Check sheet for the modelled part. Datum: model origin and axes. Units: mm. Coordinates: 2 decimals unless noted, no trailing zeros. Loops run counter-clockwise (first coordinate to the right, second up) from the corner with the lowest first, then second, coordinate; pieces in that order, holes last.
```python
from build123d import *

# Parameters (mm, degrees)
SKETCH_1_W             = 200
SKETCH_1_H             = 65
SKETCH_1_R             = 2.1
SKETCH_1_W_2           = 80
SKETCH_1_H_2           = 50
EXTRUDE_1_DEPTH        = 3
SKETCH_2_R             = 1.6
CUT_EXTRUDE_1454_DEPTH = 130.673628776
SKETCH_3_R             = 1.6
CUT_EXTRUDE_2001_DEPTH = 130.673628776
FILLET_1_R             = 10


with BuildPart() as part:
    # 草图1 → 凸台-拉伸1 (new body)
    # profile 1 of 2: a face of its own
    with BuildSketch(Plane(origin=(0, 0, 0), x_dir=(1, 0, 0), z_dir=(0, 1, 0))):
        Rectangle(SKETCH_1_W, SKETCH_1_H)
        with Locations(Location((85, -12.5, 0), (0, 0, 270))):
            Circle(SKETCH_1_R, mode=Mode.SUBTRACT)
        with Locations(Location((-85, -12.5, 0), (0, 0, 270))):
            Circle(SKETCH_1_R, mode=Mode.SUBTRACT)
        with Locations(Location((-85, 22.5, 0), (0, 0, 270))):
            Circle(SKETCH_1_R, mode=Mode.SUBTRACT)
        with Locations(Location((85, 22.5, 0), (0, 0, 270))):
            Circle(SKETCH_1_R, mode=Mode.SUBTRACT)
    # profile 2 of 2: a face of its own
    with BuildSketch(Plane(origin=(0, 0, 0), x_dir=(1, 0, 0), z_dir=(0, 1, 0))):
        with Locations((0, -57.5)):
            Rectangle(SKETCH_1_W_2, SKETCH_1_H_2)
    extrude(amount=EXTRUDE_1_DEPTH)

    # 草图2 → Cut-Extrude 1454 (cut, through all)
    with BuildSketch(Plane(origin=(0, 3, 0), x_dir=(1, 0, 0), z_dir=(0, 1, 0))):
        with Locations(Location((-60, 17.5, 0), (0, 0, 270))):
            Circle(SKETCH_2_R)
        with Locations(Location((-60, -17.5, 0), (0, 0, 270))):
            Circle(SKETCH_2_R)
        with Locations(Location((60, -17.5, 0), (0, 0, 270))):
            Circle(SKETCH_2_R)
        with Locations(Location((60, 17.5, 0), (0, 0, 270))):
            Circle(SKETCH_2_R)
    extrude(amount=-CUT_EXTRUDE_1454_DEPTH, mode=Mode.SUBTRACT)

    # 草图3 → Cut-Extrude 2001 (cut, through all)
    with BuildSketch(Plane(origin=(0, 3, 0), x_dir=(1, 0, 0), z_dir=(0, 1, 0))):
        with Locations(Location((-22.773937698, -58.5, 0), (0, 0, 270))):
            Circle(SKETCH_3_R)
        with Locations(Location((24.226062302, -58.5, 0), (0, 0, 90))):
            Circle(SKETCH_3_R)
        with Locations(Location((24.226062302, -76.5, 0), (0, 0, 270))):
            Circle(SKETCH_3_R)
        with Locations(Location((-22.773937698, -76.5, 0), (0, 0, 90))):
            Circle(SKETCH_3_R)
        with Locations(Location((-6.273937698, -59.5, 0), (0, 0, 270))):
            Circle(SKETCH_3_R)
        with Locations(Location((7.726062302, -59.5, 0), (0, 0, 90))):
            Circle(SKETCH_3_R)
        with Locations(Location((7.726062302, -75.5, 0), (0, 0, 270))):
            Circle(SKETCH_3_R)
        with Locations(Location((-6.273937698, -75.5, 0), (0, 0, 90))):
            Circle(SKETCH_3_R)
    extrude(amount=-CUT_EXTRUDE_2001_DEPTH, mode=Mode.SUBTRACT)

    # 圆角1
    fillet_1_edges = [part.edges().sort_by_distance(p)[0] for p in [
        (40, 1.5, 32.5),
        (-40, 1.5, 32.5),
    ]]
    fillet(fillet_1_edges, radius=FILLET_1_R)


solid = part.part
```
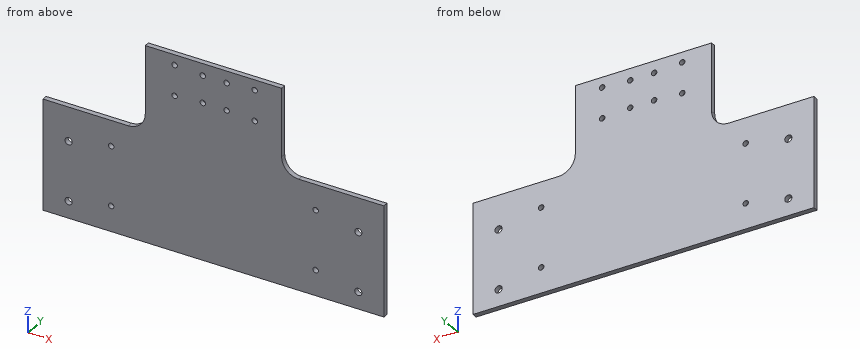
1) Section check C-C on y = 1.75. Give the number of separate pieces and of enclosed holes in the cut face, plus the area to 3 significant figures.
Answer sheet:
separate pieces: 1
enclosed holes: 16
area: 16,900 mm2
2) Section check D-D on x = 81. Enter the section's corners in (y, z).
Answer sheet:
outline: (0, -32.5) - (3, -32.5) - (3, 32.5) - (0, 32.5) - close
3) Section check B-B on z = 12.5. Enter the section's corners in (x, y).
Answer sheet:
outline: (-100, 0) - (-87.1, 0) - (-87.1, 3) - (-100, 3) - close; (-82.9, 0) - (82.9, 0) - (82.9, 3) - (-82.9, 3) - close; (87.1, 0) - (100, 0) - (100, 3) - (87.1, 3) - close
4) Scan lines: line 1 (X direction, y = 1.15, z = 12.5); line 2 (X direction, y = 1.85, z = 58.5); line 3 (X direction, y = 1.45, z = 75.5). Record each from-to range of solid material in increasing order.
Answer sheet:
line 1: x = -100 to -87.1, -82.9 to 82.9, 87.1 to 100
line 2: x = -40 to -24.37, -21.17 to -7.52, -5.02 to 6.48, 8.98 to 22.63, 25.83 to 40
line 3: x = -40 to -24.02, -21.52 to -7.87, -4.67 to 6.13, 9.33 to 22.98, 25.48 to 40
5) Section check A-A on x = -85. Enter the section's corners in (y, z).
Answer sheet:
outline: (0, -32.5) - (3, -32.5) - (3, -24.6) - (0, -24.6) - close; (0, -20.4) - (3, -20.4) - (3, 10.4) - (0, 10.4) - close; (0, 14.6) - (3, 14.6) - (3, 32.5) - (0, 32.5) - close
6) Depth check by flat-ended pin: pin 1 (1.5 mm diameter, centred on x = -76, y = 1.5, fed in from +Z). Enter the tip coordinate at first touch or a pass-through.
Answer sheet:
pin 1: stops at z = 32.5
